Work out the finished part from the listing and answer in its coordinate system (mm). Face numbers are marked on the shaded views. A direction names the side the tool comes from. Round coordinates to 2 decimals unless told otherwise and drop trailing zeros. Order: outer loops, then holes, each group sorted by start corner. A loop starts at its lowest first (then second) coordinate and runs counter-clockwise, first axis right, second up. Notation, with made-up numbers: M 59.25,63 L 102.25,63 A35 cw 102.25,95 Z; hole C -31.75,-6.5 d2. An arc over 180 degrees is marked long. Answer as a JSON object with one key per item and string values. Group by question number.
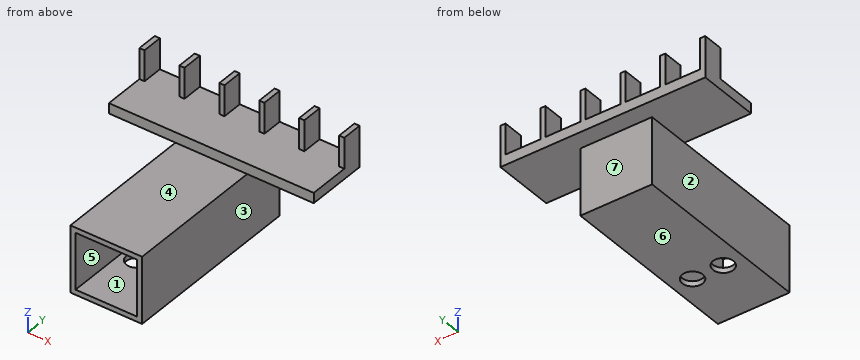
from build123d import *

# Parameters (mm, degrees)
SKETCH1_W           = 127
SKETCH1_H           = 38.1
BOSS_EXTRUDE1_DEPTH = 6.35
SKETCH2_W           = 3.175
SKETCH2_H           = 12.7
BOSS_EXTRUDE2_DEPTH = 19.05
SKETCH3_W           = 44.45
SKETCH3_H           = 114.3
BOSS_EXTRUDE3_DEPTH = 41.275
SKETCH4_W           = 38.1
SKETCH4_H           = 34.925
CUT_EXTRUDE1_DEPTH  = 50.8
SKETCH5_R           = 6.35
CUT_EXTRUDE2_DEPTH  = 23.8125


with BuildPart() as part:
    # Sketch1 → Boss-Extrude1 (new body)
    with BuildSketch(Plane.XY):
        with Locations((63.5, 19.05)):
            Rectangle(SKETCH1_W, SKETCH1_H)
    extrude(amount=BOSS_EXTRUDE1_DEPTH)

    # Sketch2 → Boss-Extrude2 (add)
    with BuildSketch(Plane.XY.offset(6.35)):
        with Locations((26.3525, 31.75)):
            Rectangle(SKETCH2_W, SKETCH2_H)
        with Locations((1.5875, 31.75)):
            Rectangle(SKETCH2_W, SKETCH2_H)
        with Locations((51.1175, 31.75)):
            Rectangle(SKETCH2_W, SKETCH2_H)
        with Locations((75.8825, 31.75)):
            Rectangle(SKETCH2_W, SKETCH2_H)
        with Locations((100.6475, 31.75)):
            Rectangle(SKETCH2_W, SKETCH2_H)
        with Locations((125.4125, 31.75)):
            Rectangle(SKETCH2_W, SKETCH2_H)
    extrude(amount=BOSS_EXTRUDE2_DEPTH)

    # Sketch3 → Boss-Extrude3 (add)
    with BuildSketch(Plane(origin=(0, 0, 0), x_dir=(-1, 0, 0), z_dir=(0, 0, -1))):
        with Locations((-63.5, -30.1625)):
            Rectangle(SKETCH3_W, SKETCH3_H)
    extrude(amount=BOSS_EXTRUDE3_DEPTH)

    # Sketch4 → Cut-Extrude1 (cut)
    with BuildSketch(Plane.XZ.offset(87.3125)):
        with Locations((63.5, -20.6375)):
            Rectangle(SKETCH4_W, SKETCH4_H)
    extrude(amount=-CUT_EXTRUDE1_DEPTH, mode=Mode.SUBTRACT)

    # Sketch5 → Cut-Extrude2 (cut)
    with BuildSketch(Plane(origin=(0, 0, -41.275), x_dir=(-1, 0, 0), z_dir=(0, 0, -1))):
        with Locations((-73.025, -49.2125)):
            Circle(SKETCH5_R)
        with Locations((-53.975, -49.2125)):
            Circle(SKETCH5_R)
    extrude(amount=-CUT_EXTRUDE2_DEPTH, mode=Mode.SUBTRACT)


solid = part.part
Item 1: A tool of negligible diameter and unlimited length cuts with its end or side. For the marked faces 5, 6 and 7, from which of +Z, -Z, +X, -X, +Y, -Y can it reach the whole face along a straight path? Write none if from no direction.
Item 2: Find section A-A (z = 14). Give the vertices of the cut face in (x, y) (3 decimals).
Item 3: Consider L1, parallel to X at y = -47, z = -36 (3 decimals); L2, parallel to Z at x = 67.5, y = -43.5 (3 decimals); L3, parallel to Z at x = 11, y = 12.5. Determine where each line is inside the solid, lowest interval first.
Item 4: Each of these flat-tipped pins is pushed along its axis until it touches: pin 1 (3.5 mm diameter, centred on x = 26, z = 12.5, fed in from -Y); pin 2 (20.5 mm diameter, centred on y = -31, z = -13, fed in from +X) (3 decimals); pin 3 (3 mm diameter, centred on x = 38, y = 19, fed in from +Z); pin 4 (2 mm diameter, centred on y = 3.5, z = 9, fed in from +X). Where does it stop, or does it pass through?
Item 5: Find section B-B (y = -77). Give the vertices of the cut face in (x, z) (3 decimals), and give its area (3 significant figures).
Item 6: The mould has two halves that part along X. Classify the marked faces 1, 2, 3 and 4: +X half, -X half, draft (parallel to the pull), parting line (faces both ways), or undercut.
Item 7: Find section D-D (y = 4.5). Give the vertices of the cut face in (x, z) (3 decimals).
Responses:
{
 "1": {"face 5": "-Y", "face 6": "-Z, +X, -X, +Y, -Y", "face 7": "-Z, +X, -X, +Y"},
 "2": {"outline": "M 0,25.4 L 3.175,25.4 L 3.175,38.1 L 0,38.1 Z; M 24.765,25.4 L 27.94,25.4 L 27.94,38.1 L 24.765,38.1 Z; M 49.53,25.4 L 52.705,25.4 L 52.705,38.1 L 49.53,38.1 Z; M 74.295,25.4 L 77.47,25.4 L 77.47,38.1 L 74.295,38.1 Z; M 99.06,25.4 L 102.235,25.4 L 102.235,38.1 L 99.06,38.1 Z; M 123.825,25.4 L 127,25.4 L 127,38.1 L 123.825,38.1 Z"},
 "3": {"L1": "x = 41.275 to 44.45, 82.55 to 85.725", "L2": "z = -41.275 to -38.1, -3.175 to 0", "L3": "z = 0 to 6.35"},
 "4": {"pin 1": "stops at y = 25.4", "pin 2": "stops at x = 85.725", "pin 3": "stops at z = 6.35", "pin 4": "passes through"},
 "5": {"outline": "M 41.275,-41.275 L 85.725,-41.275 L 85.725,0 L 41.275,0 Z; hole M 44.45,-38.1 L 82.55,-38.1 L 82.55,-3.175 L 44.45,-3.175 Z", "area": "504 mm^2"},
 "6": {"face 1": "undercut", "face 2": "-X half", "face 3": "+X half", "face 4": "draft"},
 "7": {"outline": "M 0,0 L 41.275,0 L 41.275,-41.275 L 85.725,-41.275 L 85.725,0 L 127,0 L 127,6.35 L 0,6.35 Z"}
}
